Source: CAD feature listing. Evaluate the final solid. Frame: model axes, mm. Face numbers are marked on the shaded views. A direction names the side the tool comes from. Give positions to 0.01 mm unless a question says otherwise; leave off trailing zeros. Write each loop counter-clockwise with the first axis right and the second up, starting at its lowest first coordinate (ties: lowest second). Pieces come first, ordered by that corner, then holes. Notation, with made-up numbers: (-14, -4.5) -> (24, -4.5) arc R15 cw to (24, 6.5) -> close; hole circle Ø3 at (46.5, -20). An arc over 180 degrees is marked (long way). Write item = value, one per line.
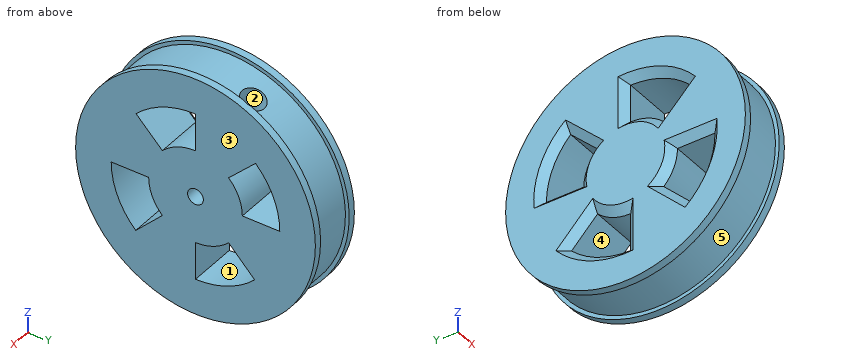
Autodesk Inventor part; units mm, degrees
ref_plane "РабПлоскость3" through (2, 0, 0) normal (1, 0, 0) x (0, 1, 0)
ref_plane "XZ Plane" through (0, 0, 0) normal (0, 1, 0) x (-1, 0, 0)
ref_plane "XY Plane" through (0, 0, 0) normal (0, 0, 1) x (1, 0, 0)
sketch "Эскиз1" plane through (0, 0, 0) normal (1, 0, 0) x (0, 1, 0)
  circle A0 centre (0, 0) radius 33
  circle A1 centre (0, 0) radius 27.5
  line L0 (27.5, 0) -> (12.5, 0)
  line L1 (0, 27.5) -> (0, 12.5)
  arc A2 (0, -12.5) -> (12.5, 0) centre (0, 0) ccw
  arc A3 (-12.5, 0) -> (0, -12.5) centre (0, 0) ccw
  arc A4 (0, 12.5) -> (-12.5, 0) centre (0, 0) ccw
  arc A5 (12.5, 0) -> (0, 12.5) centre (0, 0) ccw
  line L2 (27.5, 0) -> (22.5, 0)
  line L3 (0, -27.5) -> (0, -22.5)
  line L4 (27.5, 0) -> (22.5, 0)
  line L5 (0, 27.5) -> (0, 22.5)
  line L6 (-27.5, 0) -> (-22.5, 0)
  circle A6 centre (0, 0) radius 22.5
  line L7 (-8.8388, -8.8388) -> (-15.9436, -15.8761)
  line L8 (-12.5, 0) -> (-22.5, 0)
  line L9 (-8.8388, 8.8388) -> (-15.8761, 15.9436)
  line L10 (8.8388, 8.8388) -> (16.0277, 15.7912)
  line L11 (12.5, 0) -> (22.5, 0)
  line L12 (0, 12.5) -> (0, 22.5)
  line L13 (8.8388, -8.8388) -> (15.7912, -16.0277)
  line L14 (0, -22.5) -> (0, -12.5)
  circle A7 centre (0, 0) radius 27.5
  circle A8 centre (0, 0) radius 32
  point P0 (-27.5, 0)
  point P1 (0, 22.5)
  point P2 (0, 22.5)
  point P3 (-22.5, 0)
  point P4 (-22.5, 0)
  dimension "d2" = 15
  dimension "d3" = 15
  dimension "d4" = 15
  dimension "d5" = 15
  dimension "d21" = 5
  dimension "d22" = 5
  dimension "d25" = 360
  dimension "d67" = 64
extrude "Выдавливание1" add sketch "Эскиз1" along normal blind 15 contours L0 A6 L1 A1 | A1 L3 A6 L0 | L1 A6 L6 A1 | A1 L6 A6 L3 | A6 L13 A2 L0 | L0 A5 L10 A6 | A6 L10 A5 L1 | L1 A4 L9 A6 | L14 A2 L13 A6 | A6 L7 A3 L14 | A2 A3 A4 A5 | L8 A3 L7 A6 | A6 L9 A4 L8 | A8
sketch "Эскиз5" plane through (15, 0, 0) normal (1, 0, 0) x (0, 0, -1)
  point P0 (0, 0)
extrude "Выдавливание3" cut sketch "Эскиз1" along normal blind 15 contours L0 A5 L10 A6 | L1 A4 L9 A6 | L14 A2 L13 A6 | L8 A3 L7 A6
sketch "Эскиз6" plane through (15, 0, 0) normal (1, 0, 0) x (0, 0, -1)
  circle A0 centre (0, 0) radius 11.25
  arc A1 (0, 12.5) -> (-8.8388, 8.8388) centre (0, 0) ccw
  arc A2 (0, 12.5) -> (-8.8388, 8.8388) centre (0, 0) ccw
  line L0 (0, 0) -> (-3.0615, 7.391) construction
  circle A3 centre (-3.0615, 7.391) radius 1.5
  circle A4 centre (-7.391, -3.0615) radius 1.5
  circle A5 centre (3.0615, -7.391) radius 1.5
  circle A6 centre (7.391, 3.0615) radius 1.5
  arc A7 (-3.0615, 7.391) -> (-7.391, -3.0615) centre (0, 0) ccw
  line L1 (-8.8388, 8.8388) -> (-22.3952, 22.8573) construction
  circle A8 centre (0, 0) radius 32 construction
  line L2 (-8.8388, 8.8388) -> (10.6622, 8.8388) construction
  arc A9 (-22.3952, 22.8573) -> (-32, 0) centre (0, 0) ccw construction
  line L3 (-29.5012, 12.3966) -> (-7.391, 3.0615)
  dimension "d31" = 22.5
  dimension "d72" = 8
  dimension "d74" = 3
  dimension "d77" = 360
  dimension "d79" = 134.04
extrude "Выдавливание4" [suppressed]
extrude "Выдавливание5" cut sketch "Эскиз6" against normal blind 12 contours A3 | A4 | A0 | A5 | A6
extrude "Выдавливание6" [suppressed]
chamfer "Фаска2" distance 2 angle 45 1 edges at (0, -12.3912, -12.3575)
chamfer "Фаска3" distance 2 angle 45 15 edges at (0, -20.7964, -8.5883) (0, -17.5, 0) (0, -11.5485, -4.7835) (0, 0, -17.5) (0, 8.5331, -20.8191) (0, 12.315, -12.4333) (0, 4.7835, -11.5485) (0, 17.5, 0) (0, 11.5485, 4.7835) (0, 20.8191, 8.5331) (0, 12.4333, 12.315) (0, 0, 17.5) (0, -4.7835, 11.5485) (0, -12.3575, 12.3912) (0, -8.5883, 20.7964)
ref_plane "РабПлоскость3" through (2, 0, 0) normal (1, 0, 0) x (0, 1, 0)
sketch "Эскиз10" plane through (2, 0, 0) normal (1, 0, 0) x (0, 1, 0)
  circle A0 centre (0, 0) radius 26.5
  circle A1 centre (0, 0) radius 27.5
  circle A2 centre (0, 0) radius 26.5
  dimension "d66" = 53
sketch "Эскиз11" plane through (0, 0, 0) normal (-1, 0, 0) x (0, 0, 1)
  circle A0 centre (0, 0) radius 31
  circle A1 centre (0, 0) radius 32
  dimension "d68" = 62
extrude "Выдавливание9" cut sketch "Эскиз11" against normal blind 11 from surface at -2
sketch "Эскиз12" plane through (15, 0, 0) normal (1, 0, 0) x (0, 0, -1)
  circle A0 centre (0, 0) radius 32
  arc A1 (0, 12.5) -> (-8.8388, 8.8388) centre (0, 0) ccw
  line L0 (-8.8388, 8.8388) -> (-22.3952, 22.8573)
  circle A2 centre (0, 0) radius 32
  line L1 (-8.8388, 8.8388) -> (10.6622, 8.8388) construction
  point P0 (0, 0)
  point P1 (-32, 0)
  dimension "d85" = 134.04
ref_plane "РабПлоскость4" through (15, 12.3966, 29.5012) normal (0, 0.3874, 0.9219) x (-1, 0, 0)
sketch "Эскиз14" plane through (15, 12.3966, 29.5012) normal (0, 0.3874, 0.9219) x (-1, 0, 0)
  line L0 (0, -11.25) -> (0, 11.25)
  line L1 (0, 0) -> (5, 0)
  circle A0 centre (5, 0) radius 3.2
  circle A1 centre (5, 0) radius 1.25
  point P0 (15, 0)
  point P1 (8, 0)
  dimension "d95" = 5
  dimension "d96" = 6.4
  dimension "d99" = 2.5
extrude "Выдавливание11" [suppressed]
sketch "Эскиз15" plane through (3, 0, 0) normal (1, 0, 0) x (0, 0, -1)
  circle A0 centre (0, 0) radius 2
  dimension "d90" = 4
sketch "Эскиз16" plane through (3, 0, 0) normal (1, 0, 0) x (0, 0, -1)
  circle A0 centre (0, 0) radius 3.5
  circle A1 centre (0, 0) radius 2
  dimension "d91" = 7
  dimension "d92" = 4
extrude "Выдавливание12" add sketch "Эскиз16" along normal blind 12
ref_plane "РабПлоскость6" through (15, 1.3559, 3.2267) normal (0, 0.3874, 0.9219) x (-1, 0, 0)
extrude "Выдавливание14" cut sketch "Эскиз14" along normal blind 16 from surface at -28.5 contours A1
sketch "Эскиз18" plane through (15, 0, 0) normal (1, 0, 0) x (0, 0, -1)
  circle A0 centre (0, 0) radius 3.5
  circle A1 centre (0, 0) radius 3.5
  circle A2 centre (0, 0) radius 11.25
extrude "Выдавливание15" add sketch "Эскиз18" against normal blind 12
sketch "Эскиз19" plane through (15, 0, 0) normal (1, 0, 0) x (0, 0, -1)
  circle A0 centre (0, 0) radius 2.1
  dimension "d108" = 4.2
extrude "Выдавливание17" cut sketch "Эскиз19" against normal blind 12
extrude "Выдавливание18" cut sketch "Эскиз14" against normal blind 13 contours A1 | A0
extrude "Выдавливание19" cut sketch "Эскиз14" against normal blind 31 contours A1
properties part number "колеса прототип"
(1) Section query B-B (x = 9.5). Return loops of the section in (y, z).
Values follow:
outline = (-0.37, 2.07) -> (6.3, 17.96) -> (4.45, 18.74) -> (9.03, 29.65) arc R31 ccw (long way) to (14.86, 27.21) -> (10.27, 16.29) -> (8.42, 17.07) -> (1.74, 1.18) arc R2.1 cw (long way) to start; hole (-22.5, 0) arc R22.5 ccw to (-15.94, -15.88) -> (-8.84, -8.84) arc R12.5 cw to (-12.5, 0) -> close; hole (-15.88, 15.94) -> (-8.84, 8.84) arc R12.5 cw to (0, 12.5) -> (0, 22.5) arc R22.5 ccw to start; hole (0, -22.5) arc R22.5 ccw to (15.79, -16.03) -> (8.84, -8.84) arc R12.5 cw to (0, -12.5) -> close; hole (8.84, 8.84) arc R12.5 cw to (12.5, 0) -> (22.5, 0) arc R22.5 ccw to (16.03, 15.79) -> close
(2) Section query C-C (y = 25.5). Return loops of the section in (x, z), plus the area to 3 significant figures.
Values follow:
outline = (0, -19.33) -> (2, -19.33) -> (2, -17.63) -> (13, -17.63) -> (13, -19.33) -> (15, -19.33) -> (15, 19.33) -> (13, 19.33) -> (13, 17.63) -> (2, 17.63) -> (2, 19.33) -> (0, 19.33) -> close
area = 542 mm2
(3) Pull-direction query (Y, two-part tool) for the marked faces 3, 4 and 5; classes: pulls with the +Y half, pulls with the -Y half, needs draft (parallel to the pull), parting line crosses it, or undercut.
Values follow:
face_3 = needs draft
face_4 = undercut
face_5 = parting line crosses it
(4) Section query A-A (x = 4.5). Return loops of the section in (y, z).
Values follow:
outline = circle Ø62 at (0, 0); hole (-22.5, 0) arc R22.5 ccw to (-15.94, -15.88) -> (-8.84, -8.84) arc R12.5 cw to (-12.5, 0) -> close; hole (-15.88, 15.94) -> (-8.84, 8.84) arc R12.5 cw to (0, 12.5) -> (0, 22.5) arc R22.5 ccw to start; hole circle Ø4.2 at (0, 0); hole (0, -22.5) arc R22.5 ccw to (15.79, -16.03) -> (8.84, -8.84) arc R12.5 cw to (0, -12.5) -> close; hole (8.84, 8.84) arc R12.5 cw to (12.5, 0) -> (22.5, 0) arc R22.5 ccw to (16.03, 15.79) -> close
(5) First-contact query: pin 1 (8 mm diameter, centred on x = 13.5, y = 22.5, fed in from -Z); pin 2 (3 mm diameter, centred on x = 9.5, z = 17, fed in from -Y); pin 3 (5 mm diameter, centred on x = 5.5, y = 16, fed in from +Z); pin 4 (3 mm diameter, centred on y = 5, z = -20, fed in from -X). Flat tips, straight axial feed; report the tip coordinate or a pass-through.
Values follow:
pin_1 = -26.11
pin_2 = -26.85
pin_3 = 27.91
pin_4 = through
(6) Access query for the marked faces 1 and 2. Directions: +Z, -Z, +X, -X, +Y, -Y. A direction counts if a zero-diameter tool reaches every point of the face in a straight line with its end or side. Return the directions, or none.
Values follow:
face_1 = +X, -X
face_2 = none
(7) Material intervals for line 1 (Y direction, x = 2.75, z = 13.5); line 2 (Z direction, x = 9, y = -10); line 3 (Y direction, x = 9.75, z = 18.5), sorted ascending.
Values follow:
line_1 = -27.91 to -13.46, 0 to 13.66, 18 to 27.91
line_2 = -29.34 to -9.99, -7.5 to 10.01, 20.16 to 29.34
line_3 = -24.87 to -12.81, 0 to 5.01, 11.23 to 24.87
